Build history of the part. All positions in model axes, mm. A direction names the side the tool comes from. Round coordinates to 2 decimals unless told otherwise and drop trailing zeros. Loops run counter-clockwise (first coordinate to the right, second up) from the corner with the lowest first, then second, coordinate; pieces in that order, holes last. Notation, with made-up numbers: (-12, -33.5) - (15, -33.5) arc R24 cw to (15, -14.5) - close; hole circle Ø6 at (0, -4.5). An arc over 180 degrees is marked (long way). Put each result on its own line as item: value. Start each with the question number.
from build123d import *

# Parameters (mm, degrees)
SKETCH1_R           = 2.8
SKETCH1_W           = 3
SKETCH1_H           = 11
SKETCH1_W_2         = 11
SKETCH1_H_2         = 3
BOSS_EXTRUDE1_DEPTH = 5.5
FILLET1_R           = 10
FILLET2_R           = 10
FILLET3_R           = 10
FILLET4_R           = 10


with BuildPart() as part:
    # Sketch1 → Boss-Extrude1 (new body)
    with BuildSketch(Plane(origin=(0, 0, 0), x_dir=(1, 0, 0), z_dir=(0, 1, 0))):
        with BuildLine():
            Line((-3.5, 38.842631219), (-3.5, 36.5))
            Line((-3.5, 36.5), (3.5, 36.5))
            Line((3.5, 36.5), (3.5, 38.842631219))
            ThreePointArc((3.5, 38.842631219), (10.687785693, 37.506949182), (17.5, 34.853263836))
            Line((17.5, 34.853263836), (17.5, 17.5))
            Line((17.5, 17.5), (34.853263836, 17.5))
            ThreePointArc((34.853263836, 17.5), (37.506949182, 10.687785693), (38.842631219, 3.5))
            Line((38.842631219, 3.5), (36.5, 3.5))
            Line((36.5, 3.5), (36.5, -3.5))
            Line((36.5, -3.5), (38.842631219, -3.5))
            ThreePointArc((38.842631219, -3.5), (37.506949182, -10.687785693), (34.853263836, -17.5))
            Line((34.853263836, -17.5), (17.5, -17.5))
            Line((17.5, -17.5), (17.5, -34.853263836))
            ThreePointArc((17.5, -34.853263836), (10.687785693, -37.506949182), (3.5, -38.842631219))
            Line((3.5, -38.842631219), (3.5, -36.5))
            Line((3.5, -36.5), (-3.5, -36.5))
            Line((-3.5, -36.5), (-3.5, -38.842631219))
            ThreePointArc((-3.5, -38.842631219), (-10.687785693, -37.506949182), (-17.5, -34.853263836))
            Line((-17.5, -34.853263836), (-17.5, -17.5))
            Line((-17.5, -17.5), (-34.853263836, -17.5))
            ThreePointArc((-34.853263836, -17.5), (-37.506949182, -10.687785693), (-38.842631219, -3.5))
            Line((-38.842631219, -3.5), (-36.5, -3.5))
            Line((-36.5, -3.5), (-36.5, 3.5))
            Line((-36.5, 3.5), (-38.842631219, 3.5))
            ThreePointArc((-38.842631219, 3.5), (-37.506949182, 10.687785693), (-34.853263836, 17.5))
            Line((-34.853263836, 17.5), (-17.5, 17.5))
            Line((-17.5, 17.5), (-17.5, 34.853263836))
            ThreePointArc((-17.5, 34.853263836), (-10.687785693, 37.506949182), (-3.5, 38.842631219))
        make_face()
        with Locations(Location((0, 0, 0), (0, 0, 270))):
            Circle(SKETCH1_R, mode=Mode.SUBTRACT)
        Polygon((-8.125, 22.85), (-8.125, 20), (8.125, 20), (8.125, 22.85), (9.5, 22.85), (9.5, 28.25), (8.125, 28.25), (8.125, 31), (-8.125, 31), (-8.125, 28.25), (-9.5, 28.25), (-9.5, 22.85), align=None, mode=Mode.SUBTRACT)
        with Locations((0, 12)):
            Rectangle(SKETCH1_W, SKETCH1_H, mode=Mode.SUBTRACT)
        Polygon((22.85, 8.125), (20, 8.125), (20, -8.125), (22.85, -8.125), (22.85, -9.5), (28.25, -9.5), (28.25, -8.125), (31, -8.125), (31, 8.125), (28.25, 8.125), (28.25, 9.5), (22.85, 9.5), align=None, mode=Mode.SUBTRACT)
        with Locations((12, 0)):
            Rectangle(SKETCH1_W_2, SKETCH1_H_2, mode=Mode.SUBTRACT)
        Polygon((8.125, -22.85), (8.125, -20), (-8.125, -20), (-8.125, -22.85), (-9.5, -22.85), (-9.5, -28.25), (-8.125, -28.25), (-8.125, -31), (8.125, -31), (8.125, -28.25), (9.5, -28.25), (9.5, -22.85), align=None, mode=Mode.SUBTRACT)
        with Locations((0, -12)):
            Rectangle(SKETCH1_W, SKETCH1_H, mode=Mode.SUBTRACT)
        Polygon((-22.85, -8.125), (-20, -8.125), (-20, 8.125), (-22.85, 8.125), (-22.85, 9.5), (-28.25, 9.5), (-28.25, 8.125), (-31, 8.125), (-31, -8.125), (-28.25, -8.125), (-28.25, -9.5), (-22.85, -9.5), align=None, mode=Mode.SUBTRACT)
        with Locations((-12, 0)):
            Rectangle(SKETCH1_W_2, SKETCH1_H_2, mode=Mode.SUBTRACT)
    extrude(amount=BOSS_EXTRUDE1_DEPTH)

    # Fillet1
    fillet1_edges = [part.edges().sort_by_distance(p)[0] for p in [
        (-17.5, 2.75, 17.5),
    ]]
    fillet(fillet1_edges, radius=FILLET1_R)

    # Fillet2
    fillet2_edges = [part.edges().sort_by_distance(p)[0] for p in [
        (17.5, 2.75, 17.5),
    ]]
    fillet(fillet2_edges, radius=FILLET2_R)

    # Fillet3
    fillet3_edges = [part.edges().sort_by_distance(p)[0] for p in [
        (17.5, 2.75, -17.5),
    ]]
    fillet(fillet3_edges, radius=FILLET3_R)

    # Fillet4
    fillet4_edges = [part.edges().sort_by_distance(p)[0] for p in [
        (-17.5, 2.75, -17.5),
    ]]
    fillet(fillet4_edges, radius=FILLET4_R)


solid = part.part
Item 1: Slice it at C-C (x = 0). Give the cut face in (y, z).
Item 2: Drill centre lines: probe 1 along X at (y, z) = (1.9, 0); probe 2 along Z at (x, y) = (-3, 0.6); probe 3 along Z at (x, y) = (-29, 4.55) (3 decimals). Where is each one in solid material? Low to high. Write a range as [from, to].
Item 3: Slice it at D-D (z = -30). Give the cut face in (x, y) (3 decimals), plus the area to 3 significant figures.
Item 4: Which spindle directions (+Z, -Z, +X, -X, +Y, -Y) get a long thin tool onto all of the face, cutting with end or side? Do faces 1 (the flat face through (0, 3, 17.5)), 2 (the flat face through (3.5, 3, -38)), 3 (the flat face through (-3.5, 3, 38)), 4 (the flat face through (-38, 3, -3.5)). Say none if no direction does.
Item 5: Drop flat-ended pins along their axis: pin 1 Ø2 at (y, z) = (3, 20) entering from -X; pin 2 Ø1 at (x, y) = (-12.5, 1.5) entering from +Z; pin 3 Ø1.4 at (x, y) = (30, 1.5) entering from +Z; pin 4 Ø3 at (x, z) = (23, -20.5) entering from -Y. Give the stop position or say it passes through.
Item 6: Two-plate mould, pull along Z, no slides. Class faces 5 (the cylindrical face through (37.535, 2.712, 10.589)), 6 (the flat face through (30, 3, 8.125)), 7 (the cylindrical face through (10.589, 2.712, -37.535)), 8 (the flat face through (-17.5, 3, 31)): pulls with the +Z half, pulls with the -Z half, needs draft (parallel to the pull), parting line crosses it, or undercut.
Item 7: Slice it at B-B (z = 0). Give the cut face in (x, y), plus the area to 3 significant figures.
Item 8: Slice it at A-A (x = 21.5). Give the cut face in (y, z) (3 decimals).
Computed values:
1. outline: (0, -36.5) - (5.5, -36.5) - (5.5, -31) - (0, -31) - close; (0, -20) - (5.5, -20) - (5.5, -17.5) - (0, -17.5) - close; (0, -6.5) - (5.5, -6.5) - (5.5, -2.8) - (0, -2.8) - close; (0, 2.8) - (5.5, 2.8) - (5.5, 6.5) - (0, 6.5) - close; (0, 17.5) - (5.5, 17.5) - (5.5, 20) - (0, 20) - close; (0, 31) - (5.5, 31) - (5.5, 36.5) - (0, 36.5) - close
2. probe 1: x = [-36.5, -31], [-20, -17.5], [-6.5, -2.8], [2.8, 6.5], [17.5, 20], [31, 36.5]
2. probe 2: z = [-36.5, -31], [-20, 20], [31, 36.5]
2. probe 3: z = [-17.5, -8.125], [8.125, 17.5]
3. outline: (-17.5, 0) - (-8.125, 0) - (-8.125, 5.5) - (-17.5, 5.5) - close; (8.125, 0) - (17.5, 0) - (17.5, 5.5) - (8.125, 5.5) - close
3. area: 103 mm^2
4. face 1: +Y, -Y
4. face 2: -Z, +Y, -Y
4. face 3: +Z, +Y, -Y
4. face 4: -X, +Y, -Y
5. pin 1: stops at x = -22.23
5. pin 2: stops at z = 37.11
5. pin 3: stops at z = 17.5
5. pin 4: passes through
6. face 5: pulls with the +Z half
6. face 6: undercut
6. face 7: pulls with the -Z half
6. face 8: needs draft
7. outline: (-36.5, 0) - (-31, 0) - (-31, 5.5) - (-36.5, 5.5) - close; (-20, 0) - (-17.5, 0) - (-17.5, 5.5) - (-20, 5.5) - close; (-6.5, 0) - (-2.8, 0) - (-2.8, 5.5) - (-6.5, 5.5) - close; (2.8, 0) - (6.5, 0) - (6.5, 5.5) - (2.8, 5.5) - close; (17.5, 0) - (20, 0) - (20, 5.5) - (17.5, 5.5) - close; (31, 0) - (36.5, 0) - (36.5, 5.5) - (31, 5.5) - close
7. area: 129 mm^2
8. outline: (0, -19.5) - (5.5, -19.5) - (5.5, -8.125) - (0, -8.125) - close; (0, 8.125) - (5.5, 8.125) - (5.5, 19.5) - (0, 19.5) - close
